```python
from build123d import *

# Parameters (mm, degrees)
ESQUISSE1_W             = 90
ESQUISSE1_H             = 20
BOSS_EXTRU_1_DEPTH      = 10
ESQUISSE2_R             = 2
ENL_V_MAT_EXTRU_2_DEPTH = 94


with BuildPart() as part:
    # Esquisse1 → Boss.-Extru.1 (new body)
    with BuildSketch(Plane.XY):
        with Locations((-16.284157465, 17.946446701)):
            Rectangle(ESQUISSE1_W, ESQUISSE1_H)
    extrude(amount=BOSS_EXTRU_1_DEPTH)

    # Esquisse2 → Enlèv. mat.-Extru.2 (cut)
    with BuildSketch(Plane(origin=(0, 0, 0), x_dir=(-1, 0, 0), z_dir=(0, 0, -1))):
        with Locations((-13.715842535, 24.946446701)):
            Circle(ESQUISSE2_R)
        with Locations((-13.715842535, 10.946446701)):
            Circle(ESQUISSE2_R)
        with Locations(Location((46.284157465, 10.946446701, 0), (0, 0, 180))):
            Circle(ESQUISSE2_R)
        with Locations(Location((46.284157465, 24.946446701, 0), (0, 0, 180))):
            Circle(ESQUISSE2_R)
    extrude(amount=-ENL_V_MAT_EXTRU_2_DEPTH, mode=Mode.SUBTRACT)


solid = part.part
```
For this review, take the finished solid that the model builds, in its own axes (mm). Round coordinates to 2 decimals unless told otherwise and drop trailing zeros. Order: outer loops, then holes, each group sorted by start corner. A loop starts at its lowest first (then second) coordinate and runs counter-clockwise, first axis right, second up.
Q1. Mouldability with a two-part tool opening along X and no side actions: class faces 1 (the flat face through (-17, 18, 0)), 2 (the cylindrical face through (-48.282, 10.859, 4.93)), 3 (the cylindrical face through (-47.871, 26.163, 4.93)), 4 (the flat face through (-61.284, 18, 5)) as pulls with the +X half, pulls with the -X half, needs draft (parallel to the pull), parting line crosses it, or undercut.
Findings below:
face 1: needs draft
face 2: undercut
face 3: undercut
face 4: pulls with the -X half
Q2. Wall thickness on line 1 (X direction, y = 25.25, z = 3.25); line 2 (Y direction, x = 14.5, z = 5.75); line 3 (X direction, y = 9.25, z = 6): over which ranges is each line inside the solid? List them lowest first.
Findings below:
line 1: x = -61.28 to -48.26, -44.31 to 11.74, 15.69 to 28.72
line 2: y = 7.95 to 9.11, 12.79 to 23.11, 26.79 to 27.95
line 3: x = -61.28 to -47.34, -45.22 to 12.66, 14.78 to 28.72
Q3. We need section A-A, the plane z = 6.75. Give the boundary of the cut face in (x, y), plus the area to 3 significant figures.
Findings below:
outline: (-61.28, 7.95) - (28.72, 7.95) - (28.72, 27.95) - (-61.28, 27.95) - close; hole circle Ø4 at (-46.28, 10.95); hole circle Ø4 at (-46.28, 24.95); hole circle Ø4 at (13.72, 10.95); hole circle Ø4 at (13.72, 24.95)
area: 1,750 mm2
